from build123d import *

# Parameters (mm, degrees)
SKETCH1_R           = 4.5
SKETCH1_R_2         = 3.5
BOSS_EXTRUDE1_DEPTH = 6
FILLET1_R           = 0.5


with BuildPart() as part:
    # Sketch1 → Boss-Extrude1 (new body)
    with BuildSketch(Plane.XY):
        with Locations((-54.906305706, 0)):
            Circle(SKETCH1_R)
        with Locations((-54.906305706, 0)):
            Circle(SKETCH1_R_2, mode=Mode.SUBTRACT)
    extrude(amount=BOSS_EXTRUDE1_DEPTH)

    # Fillet1
    fillet1_edges = [part.edges().sort_by_distance(p)[0] for p in [
        (-59.406305706, 0, 0),
        (-59.406305706, 0, 6),
        (-58.406305706, 0, 0),
        (-58.406305706, 0, 6),
    ]]
    fillet(fillet1_edges, radius=FILLET1_R - 0.0001)  # a hair under: the kernel refuses the full size


solid = part.part
Geometry: final body of the model. Coordinates: model frame, mm. Give positions to 0.01 mm unless a question says otherwise; leave off trailing zeros. Write each loop counter-clockwise with the first axis right and the second up, starting at its lowest first coordinate (ties: lowest second). Pieces come first, ordered by that corner, then holes. Notation, with made-up numbers: (59.25, 4.25) - (108.25, 4.25) arc R21 ccw to (108.25, 18.25) - close; hole circle Ø3 at (-30.75, 60.5). An arc over 180 degrees is marked (long way). Return JSON: item names as keys, results as strings. Group by question number.
1) Line query: line 1 (Y direction, x = -58, z = 3.9); line 2 (Y direction, x = -57.25, z = 3.45); line 3 (X direction, y = -0.25, z = 2.5). Output: solid intervals per line, ascending.
2) Section B-B on z = 2.1. Return the cut outline in (x, y).
3) First-contact query: P1, Ø1.5, axis at y = 3, z = 3.5, coming from the +X side; P2, Ø3, axis at y = 1.5, z = 1.5, coming from the -X side; P3, Ø2, axis at y = -2.5, z = 3, coming from the -X side. Flat tips, straight axial feed; report the tip coordinate or a pass-through.
4) Mould query, pull axis X, two halves, no side actions, for faces 1 (the cylindrical face through (-51.568, 1.051, 2.965)), 2 (the cylindrical face through (-50.614, 1.352, 2.965)). Classes: released by +X, released by -X, zero draft, split by the parting line, or undercut.
Filled in:
{
 "1": {"line 1": "y = -3.27 to -1.64, 1.64 to 3.27", "line 2": "y = -3.84 to -2.6, 2.6 to 3.84", "line 3": "x = -59.4 to -58.4, -51.42 to -50.41"},
 "2": {"outline": "circle Ø9 at (-54.91, 0); hole circle Ø7 at (-54.91, 0)"},
 "3": {"P1": "stops at x = -51.01", "P2": "stops at x = -59.41", "P3": "stops at x = -59.15"},
 "4": {"face 1": "undercut", "face 2": "split by the parting line"}
}
